The model under review builds one solid part; all positions refer to its coordinate system, in mm. Face numbers are marked on the shaded views. A direction names the side the tool comes from. Give positions to 0.01 mm unless a question says otherwise; leave off trailing zeros. Loops run counter-clockwise (first coordinate to the right, second up) from the corner with the lowest first, then second, coordinate; pieces in that order, holes last. Notation, with made-up numbers: (49, 19) -> (76, 19) arc R15 cw to (76, 30) -> close; hole circle Ø11 at (74.25, -39.75). An arc over 180 degrees is marked (long way). Write each question's results on one line, items separated by ' | '. Start each with the question number.
Q1. Mouldability with a two-part tool opening along X and no side actions: class the marked faces 4, 5, 6 and 7 as released by +X, released by -X, zero draft, split by the parting line, or undercut.
Q2. We need section D-D (x = 34). Write out the cut boundary in (y, z), plus the area to 3 significant figures.
Q3. We need section B-B (x = 32.3). Write out the cut boundary in (y, z), plus the area to 3 significant figures.
Q4. Wall thickness on L1, parallel to Y at x = 32.3, z = 18.55; L2, parallel to X at y = 34.5, z = 14.85: over which ranges is each line inside the solid? List them lowest first. Write a range as [from, to].
Q5. We need section C-C (y = 39). Write out the cut boundary in (x, z).
Q6. Machinability: for the marked faces 1, 2 and 3, which of the approach directions +Z, -Z, +X, -X, +Y, -Y give a long, thin tool a straight path to every point of the face, cutting with its end or side? Answer none if there is none.
from build123d import *

# Parameters (mm, degrees)
SKETCH018_W             = 12.8
SKETCH018_H             = 6.6
SKETCH018_R             = 1
PAD004_DEPTH            = 5.7
PAD005_DEPTH            = 2.9
PAD006_DEPTH            = 2.9
BODY004_PLACEMENT_ANGLE = 90


with BuildPart() as part:
    # Sketch018 → Pad004 (new body)
    with BuildSketch(Plane.XY):
        Rectangle(SKETCH018_W, SKETCH018_H)
        with Locations((3.25, -1.7)):
            Circle(SKETCH018_R, mode=Mode.SUBTRACT)
        with BuildLine():
            ThreePointArc((-3.35, -0.7), (-4.35, -1.7), (-3.35, -2.7))
            Line((-3.35, -2.7), (-3.15, -2.7))
            ThreePointArc((-3.15, -2.7), (-2.15, -1.7), (-3.15, -0.7))
            Line((-3.15, -0.7), (-3.35, -0.7))
        make_face(mode=Mode.SUBTRACT)
    extrude(amount=PAD004_DEPTH)

    # Sketch019 (on Face11 of Pad004) → Pad005 (join)
    with BuildSketch(Plane.XY.offset(4.3)):
        with BuildLine():
            ThreePointArc((-1.35, 3.2), (-1.95, 3.8), (-2.55, 3.2))
            Line((-2.55, 3.2), (-1.35, 3.2))
        make_face()
    extrude(amount=-PAD005_DEPTH)

    # Sketch022 (on Face4 of Pad005) → Pad006 (join)
    with BuildSketch(Plane.XY.offset(4.3)):
        Polygon((-5.4, 3.3), (7.565569, 4.245522), (7.558296, 4.345257), (-5.407273, 3.399735), align=None)
    extrude(amount=-PAD006_DEPTH)


with BuildPart() as part_1:
    # Body004 placement: moved
    add(part.part.moved(Location((34, 33.95, 14))).rotate(Axis((34, 33.95, 14), (0, 0, -1)), BODY004_PLACEMENT_ANGLE))


solid = part_1.part
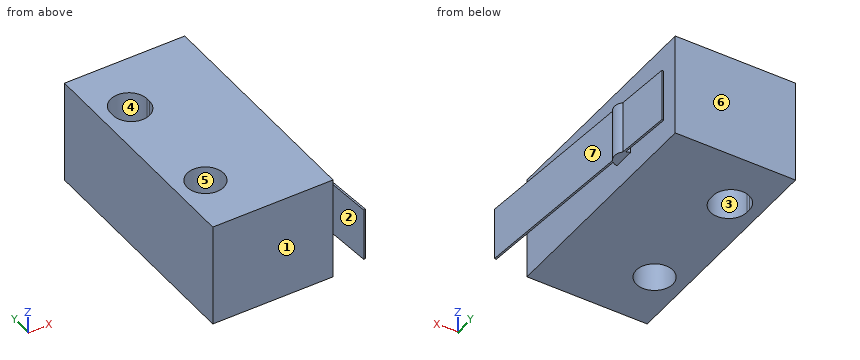
Output:
1) face 4: undercut | face 5: undercut | face 6: zero draft | face 7: released by +X
2) outline: (27.55, 14) -> (40.35, 14) -> (40.35, 19.7) -> (27.55, 19.7) -> close | area: 73.0 mm2
3) outline: (27.55, 14) -> (29.7, 14) -> (29.7, 19.7) -> (27.55, 19.7) -> close; (31.7, 14) -> (36.1, 14) -> (36.1, 19.7) -> (31.7, 19.7) -> close; (38.3, 14) -> (40.35, 14) -> (40.35, 19.7) -> (38.3, 19.7) -> close | area: 49.0 mm2
4) L1: [27.55, 29.7], [31.7, 36.1], [38.3, 40.35] | L2: [30.7, 37.3]
5) outline: (30.7, 14) -> (37.3, 14) -> (37.3, 19.7) -> (30.7, 19.7) -> close; (37.33, 15.4) -> (37.43, 15.4) -> (37.43, 18.3) -> (37.33, 18.3) -> close
6) face 1: +Z, -Z, -X, -Y | face 2: +Z, -Z, -Y | face 3: +Z, -Z
